```python
from build123d import *

# Parameters (mm, degrees)
SKETCH_1_R         = 30
EXTRUDE_1_DEPTH    = 2
HOLE_WIZARD_M3_1_D = 2.5
FILLET_1_R         = 4


with BuildPart() as part:
    # 草图1 → 凸台-拉伸1 (new body)
    with BuildSketch(Plane.XY):
        with BuildLine():
            Line((-50, 50), (-25, 50))
            Line((-25, 50), (25, 50))
            Line((25, 50), (50, 50))
            ThreePointArc((50, 50), (100, 0), (50, -50))
            Line((50, -50), (25, -50))
            Line((25, -50), (-25, -50))
            Line((-25, -50), (-50, -50))
            ThreePointArc((-50, -50), (-100, 0), (-50, 50))
        make_face()
        with Locations((-50, 0)):
            Circle(SKETCH_1_R, mode=Mode.SUBTRACT)
        with Locations((50, 0)):
            Circle(SKETCH_1_R, mode=Mode.SUBTRACT)
        with BuildLine():
            Line((-7.279981273, -20), (7.279981273, -20))
            ThreePointArc((7.279981273, -20), (14.694189797, -31.280980898), (25, -40))
            Line((25, -40), (-25, -40))
            ThreePointArc((-25, -40), (-14.694189797, -31.280980898), (-7.279981273, -20))
        make_face(mode=Mode.SUBTRACT)
        with BuildLine():
            Line((25, 40), (-25, 40))
            ThreePointArc((-25, 40), (-14.694189797, 31.280980898), (-7.279981273, 20))
            Line((-7.279981273, 20), (7.279981273, 20))
            ThreePointArc((7.279981273, 20), (14.694189797, 31.280980898), (25, 40))
        make_face(mode=Mode.SUBTRACT)
    extrude(amount=EXTRUDE_1_DEPTH)

    # M3 螺纹孔的螺纹孔钻头1 (through all)
    with Locations(Plane(origin=(-40.423695331, 35.739255573, 2), x_dir=(1, 0, 0), z_dir=(0, 0, 1))):
        with Locations((0, 0), (16.586646235, -9.576304669), (26.162950904, -26.162950904), (-19.23309471, -0.021663184), (-35.739255573, -9.576304669), (-45.315560242, -26.162950904), (126.162950904, -26.162950904), (116.586646235, -9.576304669), (100.080485372, -0.021663184), (54.684439758, -26.162950904), (64.260744427, -9.576304669), (80.847390662, 0), (80.847390662, -71.478511146), (64.260744427, -61.902206477), (54.684439758, -45.315560242), (100.080485372, -71.456847962), (116.586646235, -61.902206477), (126.162950904, -45.315560242), (-45.315560242, -45.315560242), (-35.739255573, -61.902206477), (-19.23309471, -71.456847962), (26.162950904, -45.315560242), (16.586646235, -61.902206477), (0, -71.478511146)):
            Hole(HOLE_WIZARD_M3_1_D / 2)

    # 圆角1
    fillet_1_edges = [part.edges().sort_by_distance(p)[0] for p in [
        (-7.279981273, -20, 1),
        (-25, -40, 1),
        (25, -40, 1),
        (7.279981273, -20, 1),
        (7.279981273, 20, 1),
        (25, 40, 1),
        (-25, 40, 1),
        (-7.279981273, 20, 1),
    ]]
    fillet(fillet_1_edges, radius=FILLET_1_R)


solid = part.part
```
Could you check a few things on this model? Use its own coordinates, in mm. A direction names the side the tool comes from. Coordinates: 2 decimals unless noted, no trailing zeros. Order: outer loops, then holes, each group sorted by start corner. A loop starts at its lowest first (then second) coordinate and runs counter-clockwise, first axis right, second up. Notation, with made-up numbers: M 4,-16.5 L 28,-16.5 A34 cw 28,14.5 Z; hole C 4.25,56 d10. An arc over 180 degrees is marked long. Use a Markdown table: item, result. Add a question column.
Q1. I want a section at D-D on x = -28. List the corners of the cut face in (y, z) for me.
Q2. I want a section at B-B on x = 65.5. List the corners of the cut face in (y, z) for me.
Q3. Which directions (+Z, -Z, +X, -X, +Y, -Y) give clear straight access to the entire face, cutting with the end or side of a thin tool? Please do faces 1 (the cylindrical face through (-99.988, -1.099, 0.986)), 2 (the cylindrical face through (17.35, 37.48, 1.01)).
Q4. If I drill on L1, parallel to Y at x = -3.5, z = 1.95; L2, parallel to Y at x = 15, z = 1.1; L3, parallel to X at y = 35, z = 1.6, over which ranges is the centre line in solid material (lowest first)?
Q5. I want a section at A-A on y = 0. List the corners of the cut face in (x, z) for me.
Q6. I'm going to push flat-ended pins straight in: pin 1 (2 mm diameter, centred on x = -76.16, y = 26.16, fed in from -Z); pin 2 (4 mm diameter, centred on x = -76.5, y = 14, fed in from +Z). Where does each tip first touch, or does it pass through?
Q7. I want a section at C-C on z = 1.65. Give the number of separate pieces and of enclosed holes in the cut face, then the cut area to 3 significant figures.
Q8. We'd pull the mould along Y, two halves only. Please class faces 3 (the cylindrical face through (17.35, -37.48, 1.01)), 4 (the cylindrical face through (99.988, 1.099, 0.986)), 5 (the flat face through (1, 1, 0)): pulls with the +Y half, pulls with the -Y half, needs draft (parallel to the pull), parting line crosses it, or undercut.
Checked values:
| question | item | result |
|---|---|---|
| 1 | outline | M -50,0 L -20.4,0 L -20.4,2 L -50,2 Z; M 20.4,0 L 50,0 L 50,2 L 20.4,2 Z |
| 2 | outline | M -47.54,0 L -25.69,0 L -25.69,2 L -47.54,2 Z; M 25.69,0 L 47.54,0 L 47.54,2 L 25.69,2 Z |
| 3 | face 1 | +Z, -Z, -X |
| 3 | face 2 | +Z, -Z |
| 4 | L1 | -50 to -40, -20 to 20, 40 to 50 |
| 4 | L2 | -50 to -39.76, -31.62 to -10.58, -8.57 to 8.57, 10.58 to 31.62, 39.76 to 50 |
| 4 | L3 | -85.71 to -60.68, -58.63 to -41.43, -39.42 to -17.51, 17.51 to 39.42, 41.43 to 58.63, 60.68 to 85.71 |
| 5 | outline | M -100,0 L -80,0 L -80,2 L -100,2 Z; M -20,0 L 20,0 L 20,2 L -20,2 Z; M 80,0 L 100,0 L 100,2 L 80,2 Z |
| 6 | pin 1 | through |
| 6 | pin 2 | z = 2 |
| 7 | separate pieces | 1 |
| 7 | enclosed holes | 28 |
| 7 | area | 11,000 mm² |
| 8 | face 3 | undercut |
| 8 | face 4 | parting line crosses it |
| 8 | face 5 | needs draft |
